Design review of the part built by this model. Coordinates are the model's own, in mm. Give positions to 0.01 mm unless a question says otherwise; leave off trailing zeros. Loops run counter-clockwise (first coordinate to the right, second up) from the corner with the lowest first, then second, coordinate; pieces in that order, holes last. Notation, with made-up numbers: (64.5, 23.5) -> (119.5, 23.5) arc R13 cw to (119.5, 47.5) -> close; hole circle Ø1 at (39.5, 15). An arc over 180 degrees is marked (long way). Use a Markdown table: item, result. Add a question column.
1. For pin 1 Ø12 at (y, z) = (93.5, 3.5) entering from +X; pin 2 Ø6 at (y, z) = (27, 3.5) entering from +X; pin 3 Ø4 at (x, y) = (-187.14, 1.22) entering from -Z; pin 4 Ø3 at (y, z) = (1, 2.5) entering from +X, all flat-tipped, find the tip position at first contact; note any pin that passes through.
2. Add section A-A (z = 8.75). Count the separate pieces of the cut face and the enclosed holes in it, and give its area (3 significant figures).
3. Add section B-B (y = 17.5). State the section outline as (x, z) points.
4. To check wall thickness, follow line 1 (X direction, y = -4.5, z = 12); line 2 (Y direction, x = -188, z = 16.5); line 3 (Y direction, x = -185, z = 11). State the ranges of each line that lie inside material, in increasing order.
5. Add section C-C (x = -136.5). State the section outline as (y, z) points, and give its area (3 significant figures).
Autodesk Inventor part; units mm, degrees
ref_plane "YZ Plane" through (0, 0, 0) normal (1, 0, 0) x (0, 1, 0)
ref_plane "XZ Plane" through (0, 0, 0) normal (0, 1, 0) x (-1, 0, 0)
ref_plane "XY Plane" through (0, 0, 0) normal (0, 0, 1) x (1, 0, 0)
sketch "Эскиз1" plane through (0, 0, 0) normal (0, 0, 1) x (1, 0, 0)
  circle A0 centre (0, 0) radius 165
  circle A1 centre (0, 0) radius 172.834
  line L0 (-125, 0) -> (-126.5392, 117.7261)
  line L1 (-132.7592, 119.5177) -> (-197.8467, 76.6552)
  line L2 (-165, 0) -> (-153, 0) construction
  line L3 (-134.7038, 9.8338) -> (-172.765, -2.5204)
  line L4 (-165, 0) -> (-172.8154, -2.5368)
  point P0 (-172.834, 0)
  point P1 (-126.3868, 106.0725)
  point P2 (-123, 114.4334)
  point P3 (-172.8149, -2.5694)
  dimension "d0" = 330
  dimension "d1" = 345.668
  dimension "d2" = 40
extrude "Выдавливание1" add sketch "Эскиз1" along normal blind 20 contours L3 L4 A1 L0 A0 picked at (-133.2989, 101.385)
sketch "Эскиз2" plane through (0, 0, 0) normal (0, 0, -1) x (-1, 0, 0)
  arc A0 (172.8154, -2.5368) -> (126.5392, 117.7261) centre (0, 0) ccw
  arc A1 (165, 0) -> (126.3868, 106.0725) centre (0, 0) ccw
  circle A2 centre (0, 0) radius 168.917
  line L0 (172.8154, -2.5368) -> (165, 0)
  circle A3 centre (184.6734, -6.3858) radius 2.1
  line L1 (178.0154, -4.2246) -> (172.8154, -2.5368)
  line L2 (160.1198, 6.946) -> (198.8648, -5.6302)
  line L3 (182.8662, -5.7992) -> (187.0032, 6.946)
  line L4 (178.0154, -4.2246) -> (198.192, -10.7737)
  line L5 (184.6734, -6.3858) -> (189.5243, -7.9603)
  line L6 (189.5243, -7.9603) -> (192.7095, 1.8528)
  point P0 (184.4408, -0.9483)
  point P1 (172.8109, 2.8266)
  point P2 (176.018, -3.5763)
  point P3 (182.676, -5.7374)
  point P4 (183.1424, -4.9484)
  point P5 (164.9119, 5.3905)
  point P6 (186.6708, -7.0341)
  point P7 (191.0988, -3.1094)
  dimension "d8" = 337.834
  dimension "d11" = 4.2
  dimension "d18" = 5.1
extrude "Выдавливание2" add sketch "Эскиз2" against normal up to surface (20 mm away) contours L0 A2 L2 A0 | A0 L2 L3 A3 L4 L1 | L0 A1 L2 A2 | L2 L6 L4 A3 L3 picked at (166.282, 2.7097)
sketch "Эскиз3" plane through (0, 0, 20) normal (0, 0, 1) x (1, 0, 0)
  arc A0 (-126.3868, 106.0725) -> (-165, 0) centre (0, 0) ccw
  line L0 (-126.3868, 106.0725) -> (-126.5392, 117.7261)
  arc A1 (-126.5392, 117.7261) -> (-172.8109, 2.8266) centre (0, 0) ccw
  line L1 (-191.0988, -3.1094) -> (-172.8109, 2.8266)
  line L2 (-189.5243, -7.9603) -> (-191.0988, -3.1094)
  line L3 (-186.6708, -7.0341) -> (-189.5243, -7.9603)
  arc A2 (-182.676, -5.7374) -> (-186.6708, -7.0341) centre (-184.6734, -6.3858) ccw
  line L4 (-165, 0) -> (-182.676, -5.7374)
  circle A3 centre (-184.6734, -6.3858) radius 3.1
  arc A4 (-126.5392, 117.7261) -> (-172.8109, 2.8266) centre (0, 0) ccw
  line L5 (-184.6734, -6.3858) -> (-194.1849, -9.4731)
  line L6 (-194.1849, -9.4731) -> (-195.7594, -4.6222)
  line L7 (-195.7594, -4.6222) -> (-191.0988, -3.1094)
  circle A5 centre (-184.6734, -6.3858) radius 11
  circle A6 centre (-184.6734, -6.3858) radius 9.5
  circle A7 centre (-184.6734, -6.3858) radius 6.5
  line L8 (-190.8559, -8.3925) -> (-193.7093, -9.3187)
  circle A8 centre (-192.2826, -8.8556) radius 1.6
  circle A9 centre (-182.2036, -13.995) radius 1.6
  circle A10 centre (-177.0642, -3.9159) radius 1.6
  circle A11 centre (-187.1433, 1.2234) radius 1.6
  line L9 (-192.2826, -8.8556) -> (-199.8918, -11.3255)
  line L10 (-199.8918, -11.3255) -> (-201.4663, -6.4746)
  line L11 (-201.4663, -6.4746) -> (-191.0988, -3.1094)
  line L12 (-201.4663, -6.4746) -> (-195.8644, -23.7333)
  line L13 (-172.8109, 2.8266) -> (-166.0857, -17.8924)
  line L14 (-184.6734, -6.3858) -> (-181.5861, -15.8973)
  line L15 (-165, 0) -> (-182.676, -5.7374)
  line L16 (-209.847, -25.0704) -> (-154.8396, -7.2156)
  line L17 (-201.4663, -6.4746) -> (-150.7943, 84.4559)
  line L18 (-165, 0) -> (-168.149, -11.5357)
  point P0 (-182.1957, -12.395)
  point P1 (-183.1496, -12.7046)
  point P2 (-195.5181, -4.5439)
  point P3 (-195.5997, -5.1144)
  point P4 (-193.5037, -9.8895)
  point P5 (-175.4687, -4.0356)
  point P6 (-178.5861, -4.4099)
  point P7 (-181.7249, -5.4287)
  point P8 (-187.622, -7.3428)
  point P9 (-150.9747, 84.1323)
  point P10 (-193.8045, -9.3496)
  point P11 (-196.8045, -20.837)
  point P12 (-168.149, -11.5357)
  point P13 (-171.2364, -2.0242)
  point P14 (-175.5424, -3.4219)
  point P15 (-181.1697, -15.216)
  point P16 (-182.3233, -15.5905)
  dimension "d22" = 19
  dimension "d23" = 13
  dimension "d19" = 6.2
  dimension "d20" = 10
  dimension "d21" = 22
  dimension "d24" = 3.2
  dimension "d27" = 360
  dimension "d29" = 8
  dimension "d30" = 10
  dimension "d33" = 10
extrude "Выдавливание3" add sketch "Эскиз3" against normal up to surface (20 mm away) contours A1 L1 A5 L7 L11 L17 | L11 L6 A5 L9 L10 | L1 A6 A11 L7 A5 | L13 L16 A5 L4 | L4 L18 L13 | L9 A5 L16 L12 | L7 A5 L6 | L1 A7 A11 A6 | A5 L16 L14 A9 A6 A10 L4 | L7 A6 A8 L5 L6 A5 | L9 L5 A8 A6 A9 L14 L16 A5 | A5 L6 L9 | L1 A7 A11 | A6 A11 A7 L1 L7 | L7 L2 A7 A8 A6 | L2 L5 A8 A7 | A10 A7 A9 L14 A3 L4 | A6 A9 A7 A10 | L14 A6 A9 | A9 A6 L14 | A8 A7 A9 A6 | L3 A3 L14 A9 A7 A8 L5 | A9 A7 L14 A6 | A6 L14 A7 A9 | A9 L14 A7 | L14 A9 A7
sketch "Эскиз4" plane through (0, 0, 20) normal (0, 0, 1) x (1, 0, 0)
  arc A0 (-187.622, -7.3428) -> (-181.7249, -5.4287) centre (-184.6734, -6.3858) ccw
  arc A1 (-178.5861, -4.4099) -> (-175.5424, -3.4219) centre (-177.0642, -3.9159) ccw
  circle A2 centre (-184.6734, -6.3858) radius 3.1
  circle A3 centre (-177.0642, -3.9159) radius 1.6
  point P0 (0, 0)
  point P1 (-175.5424, -3.4219)
  point P2 (-178.5861, -4.4099)
  point P3 (-181.7249, -5.4287)
  point P4 (-187.622, -7.3428)
extrude "Выдавливание4" cut sketch "Эскиз4" against normal through all
fillet "Сопряжение2" radius 10 2 edges at (-201.4663, -6.4746, 10) (-196.8045, -20.837, 10)
sketch "Эскиз5" plane through (0, 0, 20) normal (0, 0, 1) x (1, 0, 0)
  circle A0 centre (-177.0642, -3.9159) radius 1.6
  circle A1 centre (-192.2826, -8.8556) radius 1.6
  circle A2 centre (-187.1433, 1.2234) radius 1.6
  circle A3 centre (-184.6734, -6.3858) radius 3.1
  point P0 (0, 0)
properties part number "направление"
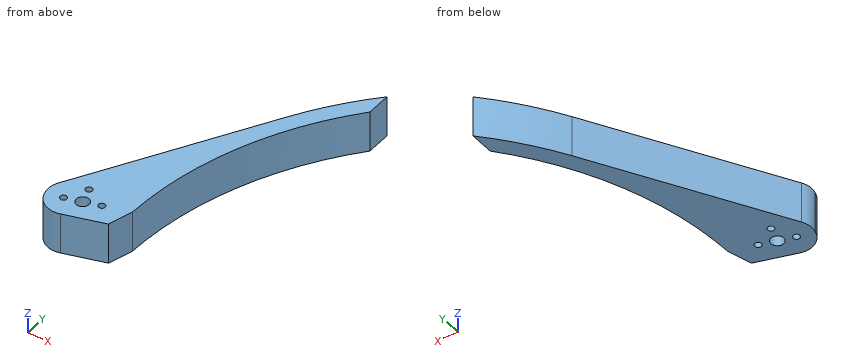
Taken from the geometry:
| question | item | result |
|---|---|---|
| 1 | pin 1 | stops at x = -131.62 |
| 1 | pin 2 | stops at x = -162.25 |
| 1 | pin 3 | stops at z = 0 |
| 1 | pin 4 | stops at x = -164.98 |
| 2 | separate pieces | 1 |
| 2 | enclosed holes | 4 |
| 2 | area | 2,140 mm^2 |
| 3 | outline | (-188.11, 0) -> (-164.07, 0) -> (-164.07, 20) -> (-188.11, 20) -> close |
| 4 | line 1 | x = -200.14 to -187.13, -182.21 to -178.55, -175.57 to -166.23 |
| 4 | line 2 | y = -17.95 to -0.13, 2.57 to 17.69 |
| 4 | line 3 | y = -17.01 to -9.47, -3.3 to 23.07 |
| 5 | outline | (92.7, 0) -> (106.02, 0) -> (106.02, 20) -> (92.7, 20) -> close |
| 5 | area | 266 mm^2 |
